Autodesk Inventor part; units mm, degrees
ref_plane "YZ Plane" through (0, 0, 0) normal (1, 0, 0) x (0, 1, 0)
ref_plane "XZ Plane" through (0, 0, 0) normal (0, 1, 0) x (-1, 0, 0)
ref_plane "XY Plane" through (0, 0, 0) normal (0, 0, 1) x (1, 0, 0)
sketch "Boceto1" plane through (0, 0, 0) normal (0, 0, 1) x (1, 0, 0)
  line L0 (0, 0) -> (300, 0)
  line L1 (300, 0) -> (300, 150)
  line L2 (300, 150) -> (0, 150)
  line L3 (0, 150) -> (0, 0)
  dimension "d0" = 150
  dimension "d1" = 300
extrude "Extrusión1" add sketch "Boceto1" along normal blind 3
sketch "Boceto3" plane through (0, 0, 3) normal (0, 0, 1) x (1, 0, 0)
  line L0 (0, 0) -> (300, 0) construction
  line L1 (300, 0) -> (300, 150) construction
  line L2 (300, 150) -> (0, 150) construction
  line L3 (0, 150) -> (0, 0) construction
  line L4 (0, 50) -> (3, 50)
  line L5 (3, 50) -> (3, 0)
  line L6 (3, 0) -> (0, 0)
  line L7 (0, 0) -> (0, 50)
  line L8 (0, 100) -> (0, 150)
  line L9 (0, 150) -> (3, 150)
  line L10 (3, 150) -> (3, 100)
  line L11 (3, 100) -> (0, 100)
  line L12 (297, 100) -> (300, 100)
  line L13 (300, 100) -> (300, 50)
  line L14 (300, 50) -> (297, 50)
  line L15 (297, 50) -> (297, 100)
  line L16 (300, 0) -> (300, 150) construction
  point P0 (300, 75)
  point P1 (300, 75)
  dimension "d15" = 3
  dimension "d16" = 50
  dimension "d19" = 100
  dimension "d24" = 3
  dimension "d25" = 50
extrude "Extrusión3" cut sketch "Boceto3" against normal blind 3
sketch "Boceto4" plane through (0, 0, 3) normal (0, 0, 1) x (1, 0, 0)
  line L0 (3, 150) -> (3, 100) construction
  line L1 (3, 100) -> (0, 100) construction
  line L2 (0, 100) -> (0, 50) construction
  line L3 (0, 50) -> (3, 50) construction
  line L4 (3, 50) -> (3, 0) construction
  line L5 (3, 0) -> (300, 0) construction
  line L6 (300, 0) -> (300, 50) construction
  line L7 (300, 50) -> (297, 50) construction
  line L8 (297, 50) -> (297, 100) construction
  line L9 (297, 100) -> (300, 100) construction
  line L10 (300, 100) -> (300, 150) construction
  line L11 (300, 150) -> (3, 150) construction
  line L12 (18, 3) -> (33, 3)
  line L13 (33, 3) -> (33, 0)
  line L14 (33, 0) -> (18, 0)
  line L15 (18, 0) -> (18, 3)
  line L16 (18, 150) -> (33, 150)
  line L17 (33, 150) -> (33, 147)
  line L18 (33, 147) -> (18, 147)
  line L19 (18, 147) -> (18, 150)
  line L20 (300, 150) -> (3, 150) construction
  line L21 (3, 0) -> (300, 0) construction
  line L22 (48, 0) -> (48, 3)
  line L23 (63, 0) -> (48, 0)
  line L24 (48, 3) -> (63, 3)
  line L25 (63, 3) -> (63, 0)
  line L26 (48, 147) -> (48, 150)
  line L27 (48, 150) -> (63, 150)
  line L28 (63, 147) -> (48, 147)
  line L29 (63, 150) -> (63, 147)
  line L30 (78, 0) -> (78, 3)
  line L31 (93, 0) -> (78, 0)
  line L32 (78, 3) -> (93, 3)
  line L33 (93, 3) -> (93, 0)
  line L34 (78, 147) -> (78, 150)
  line L35 (78, 150) -> (93, 150)
  line L36 (93, 147) -> (78, 147)
  line L37 (93, 150) -> (93, 147)
  line L38 (108, 0) -> (108, 3)
  line L39 (123, 0) -> (108, 0)
  line L40 (108, 3) -> (123, 3)
  line L41 (123, 3) -> (123, 0)
  line L42 (108, 147) -> (108, 150)
  line L43 (108, 150) -> (123, 150)
  line L44 (123, 147) -> (108, 147)
  line L45 (123, 150) -> (123, 147)
  line L46 (138, 0) -> (138, 3)
  line L47 (153, 0) -> (138, 0)
  line L48 (138, 3) -> (153, 3)
  line L49 (153, 3) -> (153, 0)
  line L50 (138, 147) -> (138, 150)
  line L51 (138, 150) -> (153, 150)
  line L52 (153, 147) -> (138, 147)
  line L53 (153, 150) -> (153, 147)
  line L54 (168, 0) -> (168, 3)
  line L55 (183, 0) -> (168, 0)
  line L56 (168, 3) -> (183, 3)
  line L57 (183, 3) -> (183, 0)
  line L58 (168, 147) -> (168, 150)
  line L59 (168, 150) -> (183, 150)
  line L60 (183, 147) -> (168, 147)
  line L61 (183, 150) -> (183, 147)
  line L62 (198, 0) -> (198, 3)
  line L63 (213, 0) -> (198, 0)
  line L64 (198, 3) -> (213, 3)
  line L65 (213, 3) -> (213, 0)
  line L66 (198, 147) -> (198, 150)
  line L67 (198, 150) -> (213, 150)
  line L68 (213, 147) -> (198, 147)
  line L69 (213, 150) -> (213, 147)
  line L70 (228, 0) -> (228, 3)
  line L71 (243, 0) -> (228, 0)
  line L72 (228, 3) -> (243, 3)
  line L73 (243, 3) -> (243, 0)
  line L74 (228, 147) -> (228, 150)
  line L75 (228, 150) -> (243, 150)
  line L76 (243, 147) -> (228, 147)
  line L77 (243, 150) -> (243, 147)
  line L78 (258, 0) -> (258, 3)
  line L79 (273, 0) -> (258, 0)
  line L80 (258, 3) -> (273, 3)
  line L81 (273, 3) -> (273, 0)
  line L82 (258, 147) -> (258, 150)
  line L83 (258, 150) -> (273, 150)
  line L84 (273, 147) -> (258, 147)
  line L85 (273, 150) -> (273, 147)
  point P0 (0, 0)
  dimension "d28" = 3
  dimension "d29" = 3
  dimension "d30" = 15
  dimension "d31" = 15
  dimension "d32" = 15
  dimension "d33" = 15
  dimension "d36" = 30
extrude "Extrusión4" cut sketch "Boceto4" against normal blind 10
properties part number "Pared2"
Geometry: final body of the model. Coordinates: model frame, mm. Give positions to 0.01 mm unless a question says otherwise; leave off trailing zeros. Write each loop counter-clockwise with the first axis right and the second up, starting at its lowest first coordinate (ties: lowest second). Pieces come first, ordered by that corner, then holes. Notation, with made-up numbers: (70.25, -29.75) -> (113.25, -29.75) arc R19 ccw to (113.25, -12.75) -> close; hole circle Ø10 at (-5, 51). An arc over 180 degrees is marked (long way). Answer as a JSON object with one key per item and string values.
1. Cut plane A-A on x = 54.5. Output: boundary loops of the cut face in (y, z), and give its area (3 significant figures).
Ans:
{"outline": "(3, 0) -> (147, 0) -> (147, 3) -> (3, 3) -> close", "area": "432 mm^2"}
2. Contact query for flat-ended pins moving along their axis: pin 1 (1 mm diameter, centred on y = 96, z = 2, fed in from +X); pin 2 (1 mm diameter, centred on y = 113.5, z = 1, fed in from -X); pin 3 (0.9 mm diameter, centred on x = 234, z = 2, fed in from +Y). Output: stop coordinate, or through.
Ans:
{"pin 1": "stops at x = 297", "pin 2": "stops at x = 3", "pin 3": "stops at y = 147"}
3. Ray query, probe 1 along X at (y, z) = (92, 2.7); probe 2 along X at (y, z) = (130, 2.6); probe 3 along Y at (x, z) = (235, 1.55). Return the intervals inside material, ascending. Write a range as from..to.
Ans:
{"probe 1": "x = 0..297", "probe 2": "x = 3..300", "probe 3": "y = 3..147"}
